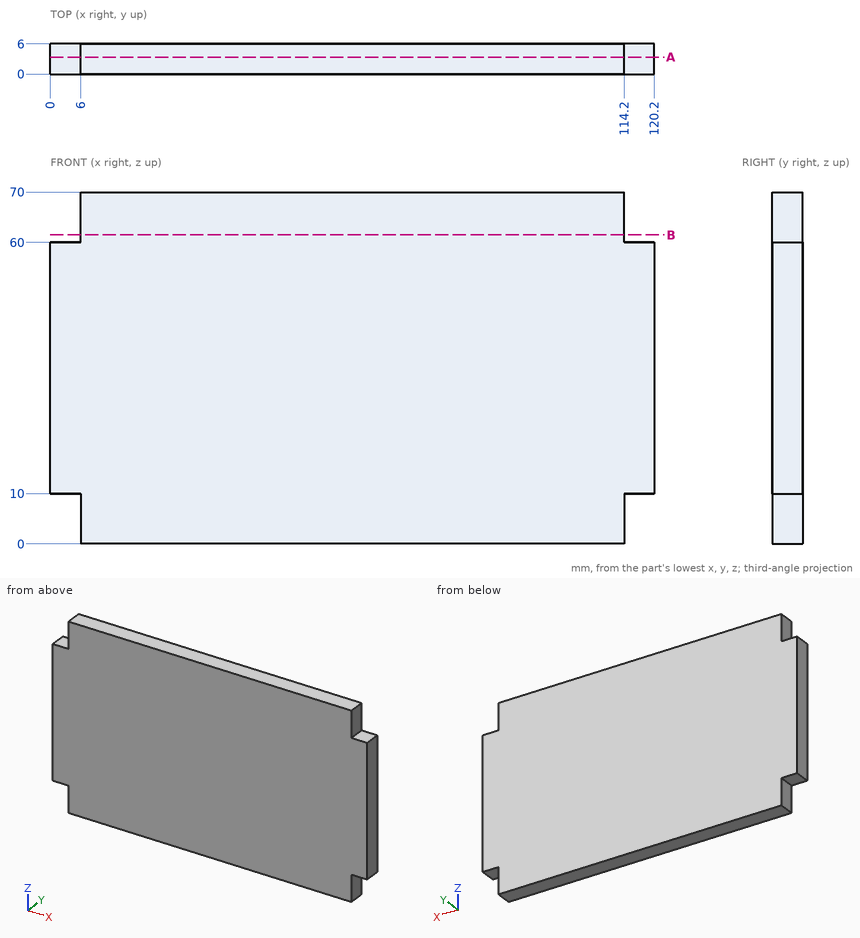
Geometry: see drawing. Coordinates: mm, zero at the bounding-box minimum. Coordinates: 2 decimals unless noted, no trailing zeros. Order: outer loops, then holes, each group sorted by start corner. A loop starts at its lowest first (then second) coordinate and runs counter-clockwise, first axis right, second up. Notation, with made-up numbers: M 26,-22.5 L 70,-22.5 A18 cw 70,-10.5 Z; hole C 59.25,71.25 d10. An arc over 180 degrees is marked long. Write each question's results on one line, items separated by ' | '. Start each with the question number.
1) Section query B-B (z = 61.5). Return the cut outline in (x, y), plus the area to 3 significant figures.
2) Line query: line 1 (X direction, y = 5.5, z = 4). Output: solid intervals per line, ascending. Write a range as from..to.
3) Section query A-A (y = 3.4). Return the cut outline in (x, z).
4) Contact query for flat-ended pins moving along their axis: pin 1 Ø1.5 at (x, y) = (81, 3) entering from -Z; pin 2 Ø3 at (x, y) = (117.5, 4.5) entering from +Z; pin 3 Ø1.8 at (y, z) = (2, 67) entering from -X; pin 4 Ø3 at (x, y) = (2, 4) entering from -Z. Output: stop coordinate, or through.
Answers:
1) outline: M 6,0 L 114.2,0 L 114.2,6 L 6,6 Z | area: 649 mm^2
2) line 1: x = 6..114.2
3) outline: M 0,10 L 6,10 L 6,0 L 114.2,0 L 114.2,10 L 120.2,10 L 120.2,60 L 114.2,60 L 114.2,70 L 6,70 L 6,60 L 0,60 Z
4) pin 1: stops at z = 0 | pin 2: stops at z = 60 | pin 3: stops at x = 6 | pin 4: stops at z = 10
